from build123d import *

# Parameters (mm, degrees)
SKETCH1_W               = 60
SKETCH1_H               = 20
SKETCH1_R               = 2.25
BOSS_EXTRUDE1_DEPTH     = 5
SKETCH2_W               = 40
SKETCH2_H               = 20
BOSS_EXTRUDE2_DEPTH     = 25
SKETCH3_R               = 2.1
CUT_EXTRUDE1_DEPTH      = 1
CUT_EXTRUDE1_DEPTH_BACK = 21
SKETCH4_R               = 3.75
CUT_EXTRUDE2_DEPTH      = 5
CUT_EXTRUDE3_DEPTH      = 4
FILLET1_R               = 7


with BuildPart() as part:
    # Sketch1 → Boss-Extrude1 (new body)
    with BuildSketch(Plane(origin=(0, 0, 0), x_dir=(1, 0, 0), z_dir=(0, 1, 0))):
        Rectangle(SKETCH1_W, SKETCH1_H)
        with Locations((-25, 0)):
            Circle(SKETCH1_R, mode=Mode.SUBTRACT)
        with Locations((25, 0)):
            Circle(SKETCH1_R, mode=Mode.SUBTRACT)
    extrude(amount=BOSS_EXTRUDE1_DEPTH)

    # Sketch2 → Boss-Extrude2 (add)
    with BuildSketch(Plane(origin=(0, 5, 0), x_dir=(1, 0, 0), z_dir=(0, 1, 0))):
        Rectangle(SKETCH2_W, SKETCH2_H)
    extrude(amount=BOSS_EXTRUDE2_DEPTH)

    # Sketch3 → Cut-Extrude1 (cut, two sides)
    with BuildSketch(Plane(origin=(0, 0, -10), x_dir=(-1, 0, 0), z_dir=(0, 0, -1))) as cut_extrude1_sk:
        with Locations((0, 20)):
            Circle(SKETCH3_R)
    extrude(amount=CUT_EXTRUDE1_DEPTH, mode=Mode.SUBTRACT)
    extrude(cut_extrude1_sk.sketch, amount=-CUT_EXTRUDE1_DEPTH_BACK, mode=Mode.SUBTRACT)

    # Sketch4 → Cut-Extrude2 (cut)
    with BuildSketch(Plane(origin=(0, 0, -10), x_dir=(-1, 0, 0), z_dir=(0, 0, -1))):
        with Locations((0, 20)):
            Circle(SKETCH4_R)
    extrude(amount=-CUT_EXTRUDE2_DEPTH, mode=Mode.SUBTRACT)

    # Sketch5 → Cut-Extrude3 (cut)
    with BuildSketch(Plane.XY.offset(10)):
        Polygon((2.078460969, 23.6), (-2.078460969, 23.6), (-4.156921938, 20), (-2.078460969, 16.4), (2.078460969, 16.4), (4.156921938, 20), align=None)
    extrude(amount=-CUT_EXTRUDE3_DEPTH, mode=Mode.SUBTRACT)

    # Fillet1
    fillet1_edges = [part.edges().sort_by_distance(p)[0] for p in [
        (-20, 30, 0),
        (20, 30, 0),
    ]]
    fillet(fillet1_edges, radius=FILLET1_R)


solid = part.part
Design review of the part built by this model. Coordinates are the model's own, in mm. A direction names the side the tool comes from. Round coordinates to 2 decimals unless told otherwise and drop trailing zeros. Write each loop counter-clockwise with the first axis right and the second up, starting at its lowest first coordinate (ties: lowest second). Pieces come first, ordered by that corner, then holes. Notation, with made-up numbers: (-37, -9.5) - (-21, -9.5) arc R23 ccw to (-21, 5.5) - close; hole circle Ø2 at (40, -37.75). An arc over 180 degrees is marked (long way). Return JSON: item names as keys, results as strings. Group by question number.
Item 1: We need section D-D on x = 0. Write out the cut boundary in (y, z), and give its area (4 significant figures).
Item 2: We need section B-B on x = -25. Write out the cut boundary in (y, z), and give its area (3 significant figures).
Item 3: The part is to be moulded in two halves that separate along Y. For faces 1 (the face through (0.81, 16.34, -7.54)), 2 (the face through (0, 30, 0)), 3 (the face through (-20, 14, 0)), say which applies: pulls with the +Y half, pulls with the -Y half, needs draft (parallel to the pull), parting line crosses it, or undercut.
Item 4: Machinability: for faces 4 (the face through (0, 16.4, 8)), 5 (the face through (20, 14, 0)), 6 (the face through (-2, 18, -5)), 7 (the face through (0, 15, 10)), 8 (the face through (-22.854, 2.465, -0.676)), which of the approach directions +Z, -Z, +X, -X, +Y, -Y give a long, thin tool a straight path to every point of the face, cutting with its end or side? Answer none if there is none.
Item 5: We need section A-A on z = 0. Write out the cut boundary in (x, y), and give its area (3 significant figures).
Item 6: We need section C-C on z = 8.25. Write out the cut boundary in (x, y).
Item 7: Insertion check: P1, Ø12, axis at x = 22.5, z = 5.5, coming from the +Y side; P2, Ø8, axis at y = 21, z = -2, coming from the -X side; P3, Ø6, axis at x = 0, y = 20, coming from the +Z side; P4, Ø3.5, axis at x = 0, y = 20, coming from the -Z side. Each pin has a flat end and moves straight along its axis. Give the tip position at first contact, or say it passes through.
Item 8: For probe 1 along X at (y, z) = (3, -0.25); probe 2 along Y at (x, z) = (0, 1.75); probe 3 along X at (y, z) = (3, -1.75), list the stretches that pass through material, from the lowest coordinate up. Write a range as [from, to].
Model answer:
{
 "1": {"outline": "(0, -10) - (16.25, -10) - (16.25, -5) - (17.9, -5) - (17.9, 6) - (16.4, 6) - (16.4, 10) - (0, 10) - close; (22.1, -5) - (23.75, -5) - (23.75, -10) - (30, -10) - (30, 10) - (23.6, 10) - (23.6, 6) - (22.1, 6) - close", "area": "487.5 mm²"},
 "2": {"outline": "(0, -10) - (5, -10) - (5, -2.25) - (0, -2.25) - close; (0, 2.25) - (5, 2.25) - (5, 10) - (0, 10) - close", "area": "77.5 mm²"},
 "3": {"face 1": "undercut", "face 2": "pulls with the +Y half", "face 3": "needs draft"},
 "4": {"face 4": "+Z", "face 5": "+Z, -Z, +X, +Y", "face 6": "-Z", "face 7": "+Z, +X, -X, +Y, -Y", "face 8": "+Y, -Y"},
 "5": {"outline": "(-30, 0) - (-27.25, 0) - (-27.25, 5) - (-30, 5) - close; (-22.75, 0) - (22.75, 0) - (22.75, 5) - (20, 5) - (20, 23) arc R7 ccw to (13, 30) - (-13, 30) arc R7 ccw to (-20, 23) - (-20, 5) - (-22.75, 5) - close; (27.25, 0) - (30, 0) - (30, 5) - (27.25, 5) - close; hole circle Ø4.2 at (0, 20)", "area": "1,220 mm²"},
 "6": {"outline": "(-30, 0) - (30, 0) - (30, 5) - (20, 5) - (20, 23) arc R7 ccw to (13, 30) - (-13, 30) arc R7 ccw to (-20, 23) - (-20, 5) - (-30, 5) - close; hole (-4.16, 20) - (-2.08, 16.4) - (2.08, 16.4) - (4.16, 20) - (2.08, 23.6) - (-2.08, 23.6) - close"},
 "7": {"P1": "stops at y = 29.06", "P2": "stops at x = -20", "P3": "stops at z = 6", "P4": "passes through"},
 "8": {"probe 1": "x = [-30, -27.24], [-22.76, 22.76], [27.24, 30]", "probe 2": "y = [0, 17.9], [22.1, 30]", "probe 3": "x = [-30, -26.41], [-23.59, 23.59], [26.41, 30]"}
}
